The model under review builds one solid part; all positions refer to its coordinate system, in mm. Face numbers are marked on the shaded views. A direction names the side the tool comes from. Coordinates: 2 decimals unless noted, no trailing zeros. Loops run counter-clockwise (first coordinate to the right, second up) from the corner with the lowest first, then second, coordinate; pieces in that order, holes last. Notation, with made-up numbers: (27, 23.5) - (32, 23.5) arc R13 ccw to (32, 35.5) - close; hole circle Ø7 at (62.25, -26.75). An arc over 180 degrees is marked (long way). Use a Markdown table: item, result. Add a question column.
1) Add section B-B, the plane y = -24.5. Give the boundary of the cut face in (x, z), and give its area (3 significant figures).
2) Add section A-A, the plane x = 0. Give the boundary of the cut face in (y, z) (3 decimals).
3) Add section C-C, the plane z = -15. Give the boundary of the cut face in (x, y) (3 decimals).
4) Add section D-D, the plane y = -3.5. Give the boundary of the cut face in (x, z), and give its area (3 significant figures).
5) Clearance check with flat-ended pins moving along their axes: pin 1 (6 mm diameter, centred on x = -8, y = -9, fed in from -Z); pin 2 (2 mm diameter, centred on y = -18.5, z = -7.5, fed in from -X); pin 3 (9.5 mm diameter, centred on x = -4, z = -5, fed in from -Y) (3 decimals). State where each tip first meets the part, or that it passes through.
6) To check wall thickness, follow L1, parallel to Y at x = -12, z = 10 (3 decimals); L2, parallel to Y at x = -9.5, z = -0.5 (3 decimals); L3, parallel to Z at x = 9, y = -26.5. State the ranges of each line that lie inside material, in increasing order. Write a range as [from, to].
7) For the marked faces 1, 2 and 3, list the 3-axis set-ups (+Z, -Z, +X, -X, +Y, -Y) from which the entire face can be reached by the end or side of a thin tool; tool diameter is ignored.
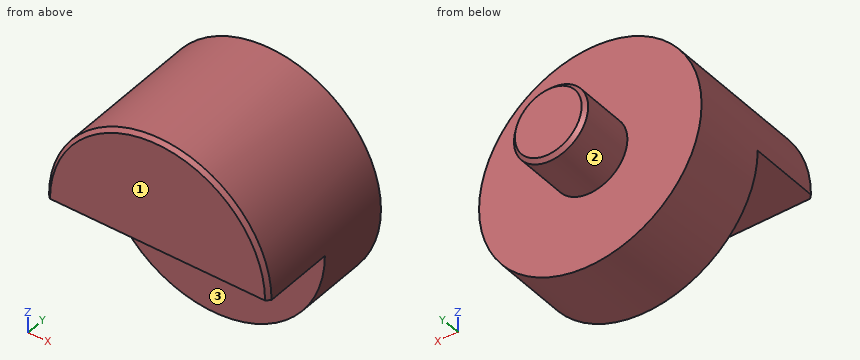
```python
from build123d import *

# Parameters (mm, degrees)
F0_R     = 19.05
F1_DEPTH = 34.925
F2_R     = 19.05
F2_R_2   = 6.35
F3_DEPTH = 9.525
F4_SIZE  = 0.635
F6_DEPTH = 12.7


with BuildPart() as f1:
    # F0 (on Front) → F1 (new body)
    with BuildSketch(Plane.XZ):
        Circle(F0_R)
    extrude(amount=F1_DEPTH)

    # F2 (on face) → F3 (cut)
    with BuildSketch(Plane(origin=(0, 0, 0), x_dir=(-1, 0, 0), z_dir=(0, 1, 0))):
        Circle(F2_R)
        Circle(F2_R_2, mode=Mode.SUBTRACT)
    extrude(amount=-F3_DEPTH, mode=Mode.SUBTRACT)

    # F4
    f4_edges = [f1.edges().sort_by_distance(p)[0] for p in [
        (6.35, 0, 0),
        (-19.05, -34.925, 0),
    ]]
    chamfer(f4_edges, length=F4_SIZE)

    # F5 (on face) → F6 (cut)
    with BuildSketch(Plane.XZ.offset(34.925)):
        with BuildLine():
            Line((-25.4, 0), (-25.4, -25.4))
            Line((-25.4, -25.4), (25.4, -25.4))
            Line((25.4, -25.4), (25.4, 0))
            Line((25.4, 0), (18.415, 0))
            ThreePointArc((18.415, 0), (0, -18.415), (-18.415, 0))
            Line((-18.415, 0), (-25.4, 0))
        make_face()
        with BuildLine():
            Line((18.415, 0), (-18.415, 0))
            ThreePointArc((-18.415, 0), (0, -18.415), (18.415, 0))
        make_face()
    extrude(amount=-F6_DEPTH, mode=Mode.SUBTRACT)


solid = f1.part
```
From the geometry:
| question | item | result |
|---|---|---|
| 1 | outline | (-19.05, 0) - (19.05, 0) arc R19.05 ccw to start |
| 1 | area | 570 mm^2 |
| 2 | outline | (-34.925, 0) - (-22.225, 0) - (-22.225, -19.05) - (-9.525, -19.05) - (-9.525, -6.35) - (-0.635, -6.35) - (0, -5.715) - (0, 5.715) - (-0.635, 6.35) - (-9.525, 6.35) - (-9.525, 19.05) - (-34.29, 19.05) - (-34.925, 18.415) - close |
| 3 | outline | (-11.743, -22.225) - (11.743, -22.225) - (11.743, -9.525) - (-11.743, -9.525) - close |
| 4 | outline | circle Ø12.7 at (0, 0) |
| 4 | area | 127 mm^2 |
| 5 | pin 1 | stops at z = -18.37 |
| 5 | pin 2 | stops at x = -17.91 |
| 5 | pin 3 | stops at y = -22.225 |
| 6 | L1 | y = [-34.925, -9.525] |
| 6 | L2 | y = [-22.225, -9.525] |
| 6 | L3 | z = [0, 16.79] |
| 7 | face 1 | +Z, -Z, +X, -X, -Y |
| 7 | face 2 | +Y |
| 7 | face 3 | -Z, +X, -X, -Y |
